Could you check a few things on this model? Use its own coordinates, in mm. Face numbers are marked on the shaded views. A direction names the side the tool comes from. Give positions to 0.01 mm unless a question says otherwise; leave off trailing zeros. Write each loop counter-clockwise with the first axis right and the second up, starting at its lowest first coordinate (ties: lowest second). Pieces come first, ordered by that corner, then holes. Notation, with made-up numbers: M 16.25,-5.5 L 42.25,-5.5 A8 cw 42.25,0.5 Z; hole C -6,48 d10. An arc over 180 degrees is marked long. Write each question's results on one line, items separated by ' | '. Start each with the question number.
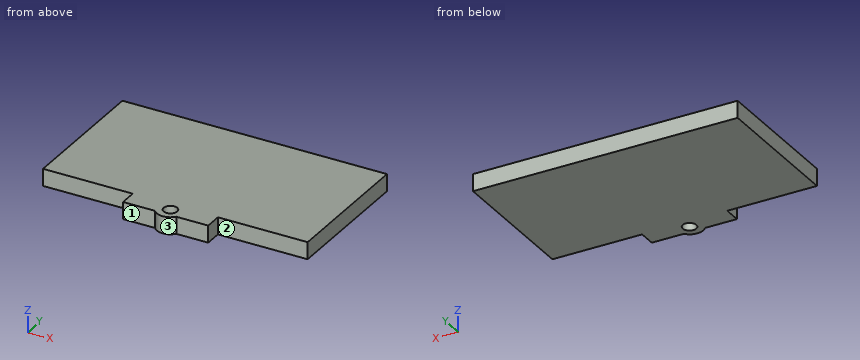
from build123d import *

# Parameters (mm, degrees)
SKETCH1_W           = 77.7
SKETCH1_H           = 41
BOSS_EXTRUDE1_DEPTH = 5
SKETCH2_W           = 25
SKETCH2_H           = 5
BOSS_EXTRUDE2_DEPTH = 5
SKETCH3_R           = 2
CUT_EXTRUDE1_DEPTH  = 5
SKETCH4_R           = 4
SKETCH4_R_2         = 2
BOSS_EXTRUDE3_DEPTH = 5


with BuildPart() as part:
    # Sketch1 → Boss-Extrude1 (new body)
    with BuildSketch(Plane.XY):
        Rectangle(SKETCH1_W, SKETCH1_H)
    extrude(amount=BOSS_EXTRUDE1_DEPTH)

    # Sketch2 → Boss-Extrude2 (add)
    with BuildSketch(Plane.XY.offset(5)):
        with Locations((0, -23)):
            Rectangle(SKETCH2_W, SKETCH2_H)
    extrude(amount=-BOSS_EXTRUDE2_DEPTH)

    # Sketch3 → Cut-Extrude1 (cut)
    with BuildSketch(Plane.XY.offset(5)):
        with Locations((-0.001489704, -23)):
            Circle(SKETCH3_R)
    extrude(amount=-CUT_EXTRUDE1_DEPTH, mode=Mode.SUBTRACT)

    # Sketch4 → Boss-Extrude3 (add)
    with BuildSketch(Plane.XY.offset(5)):
        with Locations((-0.001489704, -23)):
            Circle(SKETCH4_R)
        with Locations((-0.001489704, -23)):
            Circle(SKETCH4_R_2, mode=Mode.SUBTRACT)
    extrude(amount=-BOSS_EXTRUDE3_DEPTH)


solid = part.part
Q1. For the marked faces 1, 2 and 3, which set-ups out of +Z, -Z, +X, -X, +Y, -Y let a thin tool reach every point of the face, with its end or its side?
Q2. If we section it at C-C (x = -17): Please give me the cut outline in (y, z), plus the area to 3 significant figures.
Q3. Please list where these lines run through material, in increasing order: line 1 (Y direction, x = -18, z = 2.65); line 2 (Y direction, x = 0, z = 2.15); line 3 (Y direction, x = -5, z = 0.55). Write a range as [from, to].
Q4. If we section it at A-A (y = -23): Please give me the cut outline in (x, z), plus the area to 3 significant figures.
Q5. If we section it at B-B (z = 2.75): Please give me the cut outline in (x, y), plus the area to 3 significant figures.
Q6. I'm going to push flat-ended pins straight in: P1, Ø3, axis at x = 4, z = 1.5, coming from the -Y side; P2, Ø1.5, axis at x = -23, z = 3, coming from the -Y side; P3, Ø1.5, axis at x = -9, z = 1.5, coming from the -Y side. Where does each tip first touch, or does it pass through?
Determined:
1) face 1: +Z, -Z, -X, -Y | face 2: +Z, -Z, +X, -Y | face 3: +Z, -Z, -Y
2) outline: M -20.5,0 L 20.5,0 L 20.5,5 L -20.5,5 Z | area: 205 mm²
3) line 1: y = [-20.5, 20.5] | line 2: y = [-27, -25], [-21, 20.5] | line 3: y = [-25.5, 20.5]
4) outline: M -12.5,0 L -2,0 L -2,5 L -12.5,5 Z; M 2,0 L 12.5,0 L 12.5,5 L 2,5 Z | area: 105 mm²
5) outline: M -38.85,-20.5 L -12.5,-20.5 L -12.5,-25.5 L -3.12,-25.5 A4 ccw 3.12,-25.5 L 12.5,-25.5 L 12.5,-20.5 L 38.85,-20.5 L 38.85,20.5 L -38.85,20.5 Z; hole C 0,-23 d4 | area: 3,300 mm²
6) P1: stops at y = -26.12 | P2: stops at y = -20.5 | P3: stops at y = -25.5
